from build123d import *

# Parameters (mm, degrees)
BOSS_EXTRUDE1_DEPTH = 9.525
FILLET1_R           = 5.08
SKETCH2_R           = 4.7625
CUT_EXTRUDE1_DEPTH  = 246.132570215
BOSS_EXTRUDE2_DEPTH = 27.78125
FILLET2_R           = 5.08
FILLET3_R           = 7.62


with BuildPart() as part:
    # Sketch1 → Boss-Extrude1 (new body)
    with BuildSketch(Plane.XY):
        with BuildLine():
            Line((126.383881188, 0), (37.483881188, 0))
            ThreePointArc((37.483881188, 0), (13.166369807, 3.984360141), (-8.608104223, 15.520770598))
            Line((-8.608104223, 15.520770598), (-190.64579243, 153.796726831))
            Line((-190.64579243, 153.796726831), (-148.654110302, 153.796726831))
            Line((-148.654110302, 153.796726831), (6.755890914, 35.747180398))
            ThreePointArc((6.755890914, 35.747180398), (21.272206934, 28.056240094), (37.483881188, 25.4))
            Line((37.483881188, 25.4), (126.383881188, 25.4))
            Line((126.383881188, 25.4), (126.383881188, 0))
        make_face()
    extrude(amount=-BOSS_EXTRUDE1_DEPTH)

    # Fillet1
    fillet1_edges = [part.edges().sort_by_distance(p)[0] for p in [
        (126.383881188, 0, -4.7625),
        (126.383881188, 25.4, -4.7625),
    ]]
    fillet(fillet1_edges, radius=FILLET1_R)

    # Sketch2 → Cut-Extrude1 (cut, through all)
    with BuildSketch(Plane.XY):
        with Locations((115.271381188, 11.1125)):
            Circle(SKETCH2_R)
        with Locations((23.196381188, 12.7)):
            Circle(SKETCH2_R)
    extrude(amount=-CUT_EXTRUDE1_DEPTH, mode=Mode.SUBTRACT)

    # Sketch3 → Boss-Extrude2 (add, symmetric)
    with BuildSketch(Plane.XY.offset(-4.7625)):
        Polygon((-190.64579243, 153.796726831), (-148.654110302, 153.796726831), (-131.319590281, 153.796726831), (-123.747576859, 137.428026377), (-122.306768887, 138.09453117), (-130.304826398, 155.384226831), (-148.654110302, 155.384226831), (-190.64579243, 155.384226831), (-209.037615115, 155.384226831), (-216.380347625, 137.806207053), (-214.915512644, 137.194312678), (-207.980312451, 153.796726831), align=None)
    extrude(amount=BOSS_EXTRUDE2_DEPTH, both=True)

    # Fillet2
    fillet2_edges = [part.edges().sort_by_distance(p)[0] for p in [
        (-207.980312451, 153.796726831, -4.7625),
        (-131.319590281, 153.796726831, -4.7625),
        (-130.304826398, 155.384226831, -4.7625),
        (-209.037615115, 155.384226831, -4.7625),
    ]]
    fillet(fillet2_edges, radius=FILLET2_R)

    # Fillet3
    fillet3_edges = [part.edges().sort_by_distance(p)[0] for p in [
        (-123.027172873, 137.761278773, -32.54375),
        (-215.647930134, 137.500259865, -32.54375),
        (-123.027172873, 137.761278773, 23.01875),
        (-215.647930134, 137.500259865, 23.01875),
    ]]
    fillet(fillet3_edges, radius=FILLET3_R)


solid = part.part
Can you work these out from the model? Positions are in its coordinate system, mm. A direction names the side the tool comes from. Give positions to 0.01 mm unless a question says otherwise; leave off trailing zeros. Loops run counter-clockwise (first coordinate to the right, second up) from the corner with the lowest first, then second, coordinate; pieces in that order, holes last. Notation, with made-up numbers: M -18,-23.75 L -5,-23.75 A16 cw -5,-15.75 Z; hole C 56,-19.75 d1. An arc over 180 degrees is marked long. One line per item, written item: value. Start each with the question number.
1) If we section it at C-C, the plane x = 102: Write out the boundary of the cut face in (y, z) (3 decimals).
2) If we section it at D-D, the plane y = 54: Write out the boundary of the cut face in (x, z) (3 decimals).
3) I'm going to push flat-ended pins straight in: pin 1 (10 mm diameter, centred on x = -76.5, z = -10, fed in from +Y); pin 2 (3 mm diameter, centred on y = 106, z = -1, fed in from +X); pin 3 (7.5 mm diameter, centred on x = 115.27, y = 11.11, fed in from -Z); pin 4 (3 mm diameter, centred on x = -13.5, y = 18.5, fed in from -Z) (3 decimals). Where does each tip first touch, or does it pass through?
4) If we section it at B-B, the plane z = 6: Write out the boundary of the cut face in (x, y), and give its area (3 significant figures).
5) If I drill on line 1 (X direction, y = 12, z = -2); line 2 (Y direction, x = -195.5, z = 1); line 3 (Y direction, x = 52, z = -9), over which ranges is the centre line in solid material (lowest first)? Write a range as [from, to].
6) On a 3-axis mill with a long thin cutter (end or side, diameter ignored), from which of +Z, -Z, +X, -X, +Y, -Y can I reach the whole of each face in a straight line? I mean faces 1 (the face through (-212.14, 143.84, -4.37)), 2 (the face through (79, 25.4, -5)), 3 (the face through (-214.75, 139.61, -30.37)). Say none if no direction works.
7) Thinking about a two-plate mould opening in Y: for faces 4 (the face through (27.596, 10.876, -4.696)), 5 (the face through (-123.979, 139.846, -30.371)), 6 (the face through (-170, 154, -32.544)), which applies, +Y half, -Y half, draft (parallel to the pull), parting line (faces both ways), or undercut?
8) If we section it at A-A, the plane x = -143.5: Write out the boundary of the cut face in (y, z) (3 decimals), and give its area (3 significant figures).
Completed:
1. outline: M 0,-9.525 L 25.4,-9.525 L 25.4,0 L 0,0 Z
2. outline: M -59.265,-9.525 L -17.274,-9.525 L -17.274,0 L -59.265,0 Z
3. pin 1: stops at y = 102.77
3. pin 2: stops at x = -83.76
3. pin 3: passes through
3. pin 4: stops at z = -9.525
4. outline: M -216.38,137.81 L -214.92,137.19 L -209.28,150.67 A5.08 cw -204.6,153.8 L -134.57,153.8 A5.08 cw -129.96,150.85 L -123.75,137.43 L -122.31,138.09 L -128.94,152.44 A5.08 ccw -133.55,155.38 L -205.65,155.38 A5.08 ccw -210.34,152.26 Z
4. area: 182 mm^2
5. line 1: x = [-3.56, 18.49], [27.91, 110.59], [119.95, 126.38]
5. line 2: y = [153.8, 155.38]
5. line 3: y = [0, 25.4]
6. face 1: +Z, -Z, -Y
6. face 2: +Z, -Z, +X, +Y
6. face 3: -Z, -X, -Y
7. face 4: undercut
7. face 5: -Y half
7. face 6: draft
8. outline: M 117.985,-9.525 L 149.882,-9.525 L 149.882,0 L 117.985,0 Z; M 153.797,-32.544 L 155.384,-32.544 L 155.384,23.019 L 153.797,23.019 Z
8. area: 392 mm^2
